Build history of the part. All positions in model axes, mm. A direction names the side the tool comes from. Round coordinates to 2 decimals unless told otherwise and drop trailing zeros. Order: outer loops, then holes, each group sorted by start corner. A loop starts at its lowest first (then second) coordinate and runs counter-clockwise, first axis right, second up. Notation, with made-up numbers: (85.25, -31.5) -> (122.25, -31.5) arc R16 ccw to (122.25, -22.5) -> close; hole circle Ø7 at (-37, 21). An arc over 180 degrees is marked (long way). Answer as CSV lines item,"result". Start each with the question number.
```python
from build123d import *

# Parameters (mm, degrees)
F1_DEPTH = 854.075
F3_W     = 88.9
F3_H     = 44.45
F4_DEPTH = 127


with BuildPart() as f1:
    # F0 (on Front) → F1 (new body, symmetric)
    with BuildSketch(Plane.XZ):
        Polygon((76.2, 0), (0, 0), (0, -285.75), (76.2, -273.2717714572), align=None)
    extrude(amount=F1_DEPTH, both=True)

    # F3 (on face) → F4 (cut, symmetric)
    with BuildSketch(Plane(origin=(-45.571311316, 0, -7.4625884199), x_dir=(0, 1, 0), z_dir=(0.9868557164, 0, 0.1616038211))):
        with Locations((809.625, -259.7690209632)):
            Rectangle(F3_W, F3_H)
        with Locations((-809.625, -259.7690209632)):
            Rectangle(F3_W, F3_H)
    extrude(amount=F4_DEPTH, both=True, mode=Mode.SUBTRACT)


solid = f1.part
```
Q1. Probe L1, parallel to Y at x = 25.5, z = -271 (3 decimals); L2, parallel to Z at x = 67, y = 258; L3, parallel to Z at x = 7.5, y = 238.5. List the from-to ranges inside material, lowest first.
Q2. Slice it at B-B, the plane y = -606. Write the cut outline in (x, z).
Q3. Which spindle directions (+Z, -Z, +X, -X, +Y, -Y) get a long thin tool onto all of the face, cutting with end or side? Do faces 1 (the face through (37.567, 809.003, -234.556)), 2 (the face through (39, -765.175, -257)), 3 (the face through (39, -12, 0)). Say none if no direction does.
Q4. Flat gauge pins, fed straight in: pin 1 Ø6 at (y, z) = (467.5, -187) entering from -X; pin 2 Ø1 at (x, y) = (33.5, 526.5) entering from -Z; pin 3 Ø4 at (x, y) = (60, 655) entering from -Z; pin 4 Ø1 at (x, y) = (20, 576) entering from -Z. Where does each tip first touch, or does it go through?
Q5. Slice it at A-A, the plane x = 36. Write the cut outline in (y, z) (3 decimals).
Solutions:
1,L1,"y = -765.175 to 765.175"
1,L2,"z = -274.78 to 0"
1,L3,"z = -284.52 to 0"
2,outline,"(0, -285.75) -> (76.2, -273.27) -> (76.2, 0) -> (0, 0) -> close"
3,face 1,"-Z, +X, +Y"
3,face 2,"-Z, +X, -Y"
3,face 3,"+Z, +X, -X, +Y, -Y"
4,pin 1,"stops at x = 0"
4,pin 2,"stops at z = -280.35"
4,pin 3,"stops at z = -276.25"
4,pin 4,"stops at z = -282.56"
5,outline,"(-854.075, -234.813) -> (-765.175, -234.813) -> (-765.175, -279.855) -> (765.175, -279.855) -> (765.175, -234.813) -> (854.075, -234.813) -> (854.075, 0) -> (-854.075, 0) -> close"
